from build123d import *

# Parameters (mm, degrees)
BOSS_EXTRUDE1_DEPTH                            = 9.525
SKETCH2_W                                      = 1.89865
SKETCH2_H                                      = 43.65625
F_10_CLEARANCE_HOLE1_D                         = 5.1054
F_10_CLEARANCE_HOLE1_DEPTH                     = 11.90625
F_10_CLEARANCE_HOLE2_D                         = 5.1054
F_10_CLEARANCE_HOLE2_DEPTH                     = 11.90625
F_10_24_TAPPED_HOLE2_D                         = 3.7973
CBORE_FOR_8_SOCKET_HEAD_CAP_SCREW1_D           = 4.9149
CBORE_FOR_8_SOCKET_HEAD_CAP_SCREW1_CBORE_D     = 7.9375
CBORE_FOR_8_SOCKET_HEAD_CAP_SCREW1_CBORE_DEPTH = 16.8656
HOLE1_START                                    = 4.0894
HOLE1_OUTLINE_R                                = 1.7272
HOLE1_OUTLINE_R_2                              = 3.96875
HOLE1_OUTLINE_R_3                              = 4.7625
HOLE1_DEPTH                                    = 5.4356
HOLE1_2_OUTLINE_R                              = 1.7272
HOLE1_2_OUTLINE_R_2                            = 2.45745
HOLE1_2_OUTLINE_R_3                            = 4.7625
HOLE1_2_DEPTH                                  = 4.0894
HOLE1_3_OUTLINE_R                              = 6.35
HOLE1_3_OUTLINE_R_2                            = 4.7625
HOLE1_3_DEPTH                                  = 1.5875
F_8_32_TAPPED_HOLE2_D                          = 3.4544


# Read off the part's stored shape, not the designer's step: Hole1
with BuildPart() as part:
    # Sketch1 → Boss-Extrude1 (new body)
    with BuildSketch(Plane(origin=(0, 0, 0), x_dir=(1, 0, 0), z_dir=(0, 1, 0))):
        with BuildLine():
            Line((120.206642486, 6.011694636), (120.206642486, 17.917944636))
            Line((120.206642486, 17.917944636), (110.631837795, 17.917944636))
            ThreePointArc((110.631837795, 17.917944636), (97.981642486, 18.711694636), (110.631837795, 19.505444636))
            Line((110.631837795, 19.505444636), (120.206642486, 19.505444636))
            Line((120.206642486, 19.505444636), (120.206642486, 31.411694636))
            Line((120.206642486, 31.411694636), (-438.593357514, 31.411694636))
            Line((-438.593357514, 31.411694636), (-438.593357514, 19.505444636))
            Line((-438.593357514, 19.505444636), (-429.018552824, 19.505444636))
            ThreePointArc((-429.018552824, 19.505444636), (-416.368357514, 18.711694636), (-429.018552824, 17.917944636))
            Line((-429.018552824, 17.917944636), (-438.593357514, 17.917944636))
            Line((-438.593357514, 17.917944636), (-438.593357514, 6.011694636))
            Line((-438.593357514, 6.011694636), (37.656642486, 6.011694636))
            Line((37.656642486, 6.011694636), (37.656642486, -25.738305364))
            Line((37.656642486, -25.738305364), (94.806642486, -25.738305364))
            Line((94.806642486, -25.738305364), (94.806642486, 6.011694636))
            Line((94.806642486, 6.011694636), (120.206642486, 6.011694636))
        make_face()
    extrude(amount=BOSS_EXTRUDE1_DEPTH)

    # Sketch2 → #10-24 Tapped Hole1 (revolve, cut)
    with BuildSketch(Plane(origin=(115.444142486, 4.7625, -17.917944636), x_dir=(0, 1, 0), z_dir=(1, 0, 0))):
        with Locations((0.949325, 21.828125)):
            Rectangle(SKETCH2_W, SKETCH2_H)
    revolve(axis=Axis((115.444142486, 4.7625, -24.267944636), (0, 0, 1)), mode=Mode.SUBTRACT)

    # #10 Clearance Hole1
    with Locations(Plane(origin=(0, 0, -31.411694636), x_dir=(-1, 0, 0), z_dir=(0, 0, -1))):
        with Locations((-115.444142486, 4.7625)):
            Hole(F_10_CLEARANCE_HOLE1_D / 2, depth=F_10_CLEARANCE_HOLE1_DEPTH)

    # #10 Clearance Hole2
    with Locations(Plane(origin=(0, 0, -31.411694636), x_dir=(-1, 0, 0), z_dir=(0, 0, -1))):
        with Locations((433.830857514, 4.7625)):
            Hole(F_10_CLEARANCE_HOLE2_D / 2, depth=F_10_CLEARANCE_HOLE2_DEPTH)

    # #10-24 Tapped Hole2 (through all)
    with Locations(Plane(origin=(0, 0, -17.917944636), x_dir=(-1, 0, 0), z_dir=(0, 0, -1))):
        with Locations((433.830857514, 4.7625)):
            Hole(F_10_24_TAPPED_HOLE2_D / 2)

    # CBORE for #8 Socket Head Cap Screw1 (through all)
    with Locations(Plane(origin=(0, 0, -31.411694636), x_dir=(-1, 0, 0), z_dir=(0, 0, -1))):
        with Locations((-31.306642486, 4.7625), (-18.606642486, 4.7625), (406.843357514, 4.7625), (394.143357514, 4.7625)):
            CounterBoreHole(CBORE_FOR_8_SOCKET_HEAD_CAP_SCREW1_D / 2, CBORE_FOR_8_SOCKET_HEAD_CAP_SCREW1_CBORE_D / 2, CBORE_FOR_8_SOCKET_HEAD_CAP_SCREW1_CBORE_DEPTH)

    # Hole1 outline → Hole1 (cut)
    with BuildSketch(Plane(origin=(0, 0, 0), x_dir=(1, 0, 0), z_dir=(0, 1, 0)).offset(HOLE1_START)):
        with Locations((-3.618357514, 25.061694636)):
            Circle(HOLE1_OUTLINE_R)
        with Locations((-77.278357514, 25.061694636)):
            Circle(HOLE1_OUTLINE_R)
        with Locations((-150.938357514, 25.061694636)):
            Circle(HOLE1_OUTLINE_R)
        with Locations((-224.598357514, 25.061694636)):
            Circle(HOLE1_OUTLINE_R)
        with Locations((-298.258357514, 25.061694636)):
            Circle(HOLE1_OUTLINE_R)
        with Locations((-371.918357514, 25.061694636)):
            Circle(HOLE1_OUTLINE_R)
        with Locations((-3.618357514, 10.774194636)):
            Circle(HOLE1_OUTLINE_R_2)
        with Locations((-77.278357514, 10.774194636)):
            Circle(HOLE1_OUTLINE_R_2)
        with Locations((-150.938357514, 10.774194636)):
            Circle(HOLE1_OUTLINE_R_2)
        with Locations((-224.598357514, 10.774194636)):
            Circle(HOLE1_OUTLINE_R_2)
        with Locations((-298.258357514, 10.774194636)):
            Circle(HOLE1_OUTLINE_R_2)
        with Locations((-371.918357514, 10.774194636)):
            Circle(HOLE1_OUTLINE_R_2)
        with Locations((66.231642486, 2.836694636)):
            Circle(HOLE1_OUTLINE_R_3)
    extrude(amount=HOLE1_DEPTH, mode=Mode.SUBTRACT)

    # Hole1 2 outline → Hole1 2 (cut)
    with BuildSketch(Plane(origin=(0, 0, 0), x_dir=(1, 0, 0), z_dir=(0, 1, 0))):
        with Locations((-3.618357514, 25.061694636)):
            Circle(HOLE1_2_OUTLINE_R)
        with Locations((-77.278357514, 25.061694636)):
            Circle(HOLE1_2_OUTLINE_R)
        with Locations((-150.938357514, 25.061694636)):
            Circle(HOLE1_2_OUTLINE_R)
        with Locations((-224.598357514, 25.061694636)):
            Circle(HOLE1_2_OUTLINE_R)
        with Locations((-298.258357514, 25.061694636)):
            Circle(HOLE1_2_OUTLINE_R)
        with Locations((-371.918357514, 25.061694636)):
            Circle(HOLE1_2_OUTLINE_R)
        with Locations((-3.618357514, 10.774194636)):
            Circle(HOLE1_2_OUTLINE_R_2)
        with Locations((-77.278357514, 10.774194636)):
            Circle(HOLE1_2_OUTLINE_R_2)
        with Locations((-150.938357514, 10.774194636)):
            Circle(HOLE1_2_OUTLINE_R_2)
        with Locations((-224.598357514, 10.774194636)):
            Circle(HOLE1_2_OUTLINE_R_2)
        with Locations((-298.258357514, 10.774194636)):
            Circle(HOLE1_2_OUTLINE_R_2)
        with Locations((-371.918357514, 10.774194636)):
            Circle(HOLE1_2_OUTLINE_R_2)
        with Locations((66.231642486, 2.836694636)):
            Circle(HOLE1_2_OUTLINE_R_3)
    extrude(amount=HOLE1_2_DEPTH, mode=Mode.SUBTRACT)

    # Hole1 3 outline → Hole1 3 (cut)
    with BuildSketch(Plane(origin=(0, 0, 0), x_dir=(1, 0, 0), z_dir=(0, 1, 0))):
        with Locations((66.231642486, 2.836694636)):
            Circle(HOLE1_3_OUTLINE_R)
        with Locations((66.231642486, 2.836694636)):
            Circle(HOLE1_3_OUTLINE_R_2, mode=Mode.SUBTRACT)
    extrude(amount=HOLE1_3_DEPTH, mode=Mode.SUBTRACT)

    # #8-32 Tapped Hole2 (through all)
    with Locations(Plane(origin=(0, 0, 0), x_dir=(-1, 0, 0), z_dir=(0, -1, 0))):
        with Locations((-94.806642486, 28.236694636), (-113.856642486, 9.186694636), (432.243357514, 9.186694636), (413.193357514, 28.236694636)):
            Hole(F_8_32_TAPPED_HOLE2_D / 2)


solid = part.part
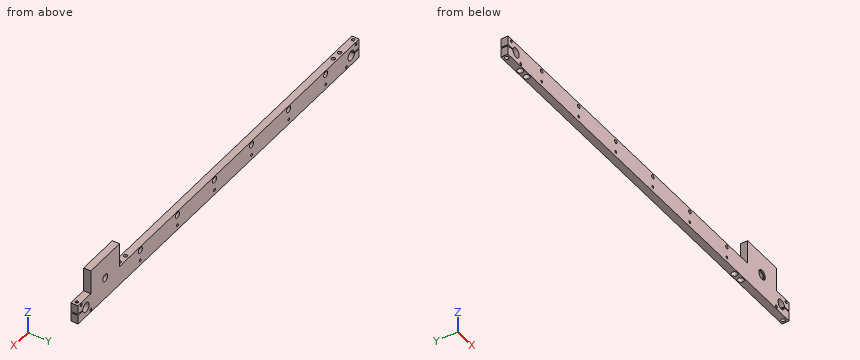
CAD build for the part. Positions are in the model's coordinates, mm. Round coordinates to 2 decimals unless told otherwise and drop trailing zeros. Write each loop counter-clockwise with the first axis right and the second up, starting at its lowest first coordinate (ties: lowest second). Pieces come first, ordered by that corner, then holes.
(1) Drop flat-ended pins along their axis: P1, Ø1, axis at x = -196, y = 3.5, coming from the +Z side; P2, Ø7.5, axis at x = -422.72, z = -18.71, coming from the +Y side; P3, Ø6.5, axis at x = -77.28, z = -10.77, coming from the +Y side; P4, Ø4, axis at x = -392.5, y = 4, coming from the -Z side. Give the stop position or say it passes through.
(2) Slice it at A-A, the plane x = -332. Write the cut outline in (y, z) (3 decimals).
(3) Slice it at B-B, the plane z = 10. Write the cut outline in (x, y) (3 decimals), and give its area (3 significant figures).
(4) Probe line 1 along Z through (x, y) = (-150.5, 9); line 2 along Z through (x, y) = (-225.5, 7.5); line 3 along Z through (x, y) = (-267.5, 1.25). List the from-to ranges inside material, lowest first.
From the geometry:
1. P1: stops at z = -6.01
1. P2: passes through
1. P3: stops at y = 4.09
1. P4: stops at z = -14.55
2. outline: (0, -31.412) - (9.525, -31.412) - (9.525, -6.012) - (0, -6.012) - close
3. outline: (37.657, 0) - (94.807, 0) - (94.807, 9.525) - (37.657, 9.525) - close
3. area: 544 mm2
4. line 1: z = -31.41 to -26.73, -23.39 to -14.72, -6.83 to -6.01
4. line 2: z = -31.41 to -26.53, -23.59 to -14.64, -6.91 to -6.01
4. line 3: z = -31.41 to -6.01
